Here's how the part is built. I have some questions about the finished solid (model axes, mm). A direction names the side the tool comes from. Coordinates: 2 decimals unless noted, no trailing zeros. Write each loop counter-clockwise with the first axis right and the second up, starting at its lowest first coordinate (ties: lowest second). Pieces come first, ordered by that corner, then holes. Notation, with made-up numbers: (81.25, -18.5) -> (103.25, -18.5) arc R26 ccw to (103.25, 12.5) -> close; hole circle Ø2 at (-36, 23). An arc over 180 degrees is marked (long way). Put each result on its own line as item: value. Start each with the question number.
Item 1: I want a section at A-A, the plane y = 0. List the corners of the cut face in (x, z) for me.
Item 2: On a 3-axis mill with a long thin cutter (end or side, diameter ignored), from which of +Z, -Z, +X, -X, +Y, -Y can I reach the whole of each face in a straight line? I mean faces 1 (the face through (105, 0, -16)), 2 (the face through (59, 6, 1)). Say none if no direction works.
Item 3: I need wall thicknesses on line 1 (Z direction, x = 99, y = 0); line 2 (X direction, y = -3.75, z = -18.5); line 3 (X direction, y = -3, z = -4). Which ranges of each line are inside material? Lowest first, please. Write a range as [from, to].
Item 4: For pin 1 (6 mm diameter, centred on y = -1, z = -13, fed in from -X), with a flat end and sliding along its axis, tell me the tip position at first contact or that it passes through.
Item 5: I want a section at C-C, the plane z = -8.5. List the corners of the cut face in (x, y) for me, then the cut area to 3 significant figures.
Item 6: I want a section at B-B, the plane x = 13. List the corners of the cut face in (y, z) for me, then the cut area to 3 significant figures.
from build123d import *

# Parameters (mm, degrees)
BOX_W        = 110
BOX_H        = 12
BOX_DEPTH    = 12
POCKET_DEPTH = 12
SKETCH001_W  = 5
SKETCH001_H  = 20
PAD_DEPTH    = 12


with BuildPart() as part:
    # Box → Box (new body)
    with BuildSketch(Plane(origin=(0, -6, -6), x_dir=(1, 0, 0), z_dir=(0, 0, 1))):
        with Locations((55, 6)):
            Rectangle(BOX_W, BOX_H)
    extrude(amount=BOX_DEPTH)

    # Sketch → Pocket (cut)
    with BuildSketch(Plane(origin=(0, -6, -6), x_dir=(1, 0, 0), z_dir=(0, -1, 0))):
        with BuildLine():
            ThreePointArc((0, 0.75), (5.25, 6), (0, 11.25))
            Line((0, 11.25), (0, 0.75))
        make_face()
    extrude(amount=-POCKET_DEPTH, mode=Mode.SUBTRACT)

    # Sketch001 → Pad (new body)
    with BuildSketch(Plane(origin=(0, -6, -6), x_dir=(1, 0, 0), z_dir=(0, -1, 0))):
        with Locations((107.5, -10)):
            Rectangle(SKETCH001_W, SKETCH001_H)
    extrude(amount=-PAD_DEPTH)


solid = part.part
Calculated:
1. outline: (0, -6) -> (105, -6) -> (105, -26) -> (110, -26) -> (110, 6) -> (0, 6) -> (0, 5.25) arc R5.25 cw to (0, -5.25) -> close
2. face 1: -Z, -X, +Y, -Y
2. face 2: +Z, -Z, +X, -X, +Y
3. line 1: z = [-6, 6]
3. line 2: x = [105, 110]
3. line 3: x = [3.4, 110]
4. pin 1: stops at x = 105
5. outline: (105, -6) -> (110, -6) -> (110, 6) -> (105, 6) -> close
5. area: 60.0 mm2
6. outline: (-6, -6) -> (6, -6) -> (6, 6) -> (-6, 6) -> close
6. area: 144 mm2
